Read the model definition and answer for the solid it produces. Units are mm, in the model's axes. A direction names the side the tool comes from. Round coordinates to 2 decimals unless told otherwise and drop trailing zeros. Order: outer loops, then holes, each group sorted by start corner. A loop starts at its lowest first (then second) coordinate and runs counter-clockwise, first axis right, second up. Notation, with made-up numbers: (18, 86) - (69, 86) arc R31 cw to (69, 120) - close; hole circle Ø2 at (57, 27.25). An arc over 180 degrees is marked (long way). Put each result on its own line as item: value. Start each with the question number.
Q1. Section A-A on x = -13.5 is taken. Give the vertices of the cut face in (y, z), then the cut area to 3 significant figures.
Q2. Find the intervals of material crossed by line 1 along Y through (x, z) = (0, 15.25); line 2 along Z through (x, y) = (14, 17); line 3 along X through (y, z) = (20, 13.75), in increasing order. Write a range as from..to.
Q3. Each of these flat-tipped pins is pushed along its axis until it touches: pin 1 Ø1.2 at (x, y) = (-6.93, -4) entering from -Z; pin 2 Ø25 at (x, y) = (11, 6.5) entering from -Z; pin 3 Ø1.5 at (x, z) = (17.5, 10.5) entering from +Y; pin 4 Ø6.5 at (x, y) = (0, 0) entering from -Z. Where does it stop, or does it pass through?
Q4. Section D-D on x = 18 is taken. Give the vertices of the cut face in (y, z).
Q5. Which of the six approach directions +Z, -Z, +X, -X, +Y, -Y give full straight-line access (tool end or side, diameter ignored) to faces 1 (the face through (-24, -24, 3)), 2 (the face through (-1.172, 8.923, 2.493)), 3 (the face through (24, -24, 14.5))?
Q6. For a pull along Y with two mould halves and no side action, classify faces 4 (the face through (0, 6, 14.5)), 5 (the face through (-11.5, 0.4, 0)), 6 (the face through (0, -25, 1)), 7 (the face through (-24, 24, 0)) as pulls with the +Y half, pulls with the -Y half, needs draft (parallel to the pull), parting line crosses it, or undercut.
Q7. Section B-B on z = 16.5 is taken. Give the vertices of the cut face in (x, y), then the cut area to 3 significant figures.
from build123d import *

# Parameters (mm, degrees)
SKETCH_W          = 50
SKETCH_H          = 50
SKETCH_R          = 9
PAD_DEPTH         = 3
SKETCH001_R       = 4
PAD001_DEPTH      = 1
PAD001_DEPTH_BACK = 14.5
SKETCH002_W       = 50
SKETCH002_H       = 50
SKETCH002_R       = 1
SKETCH002_R_2     = 3
SKETCH002_R_3     = 2
PAD002_DEPTH      = 3
FILLET_R          = 2


with BuildPart() as part:
    # Sketch → Pad (new body)
    with BuildSketch(Plane.XY):
        Rectangle(SKETCH_W, SKETCH_H)
        Circle(SKETCH_R, mode=Mode.SUBTRACT)
    extrude(amount=PAD_DEPTH)

    # Sketch001 (on Face6 of Pad) → Pad001 (join, two sides)
    with BuildSketch(Plane(origin=(0, 0, 0), x_dir=(1, 0, 0), z_dir=(0, 0, -1))) as pad001_sk:
        with Locations((-21, 21)):
            Circle(SKETCH001_R)
        with Locations((21, 21)):
            Circle(SKETCH001_R)
        with Locations((21, -21)):
            Circle(SKETCH001_R)
        with Locations((-21, -21)):
            Circle(SKETCH001_R)
    extrude(amount=PAD001_DEPTH)
    extrude(pad001_sk.sketch, amount=-PAD001_DEPTH_BACK)

    # Sketch002 (on Face25 of Pad001) → Pad002 (join)
    with BuildSketch(Plane.XY.offset(14.5)):
        Rectangle(SKETCH002_W, SKETCH002_H)
        with Locations((0, 8)):
            Circle(SKETCH002_R, mode=Mode.SUBTRACT)
        with Locations((6.928203, -4)):
            Circle(SKETCH002_R, mode=Mode.SUBTRACT)
        with Locations((-6.928203, -4)):
            Circle(SKETCH002_R, mode=Mode.SUBTRACT)
        with Locations((0, -8)):
            Circle(SKETCH002_R_2, mode=Mode.SUBTRACT)
        Circle(SKETCH002_R_3, mode=Mode.SUBTRACT)
    extrude(amount=PAD002_DEPTH)

    # Fillet
    fillet_edges = [part.edges().sort_by_distance(p)[0] for p in [
        (-9, 0, 0),
    ]]
    fillet(fillet_edges, radius=FILLET_R)


solid = part.part
Findings:
1. outline: (-25, 0) - (25, 0) - (25, 3) - (-25, 3) - close; (-25, 14.5) - (25, 14.5) - (25, 17.5) - (-25, 17.5) - close
1. area: 300 mm2
2. line 1: -25..-11, -5..-2, 2..7, 9..25
2. line 2: 0..3, 14.5..17.5
2. line 3: -24.87..-17.13, 17.13..24.87
3. pin 1: through
3. pin 2: z = 0
3. pin 3: y = 23.9
3. pin 4: z = 14.5
4. outline: (-25, 0) - (-23.65, 0) - (-23.65, -1) - (-18.35, -1) - (-18.35, 0) - (18.35, 0) - (18.35, -1) - (23.65, -1) - (23.65, 0) - (25, 0) - (25, 3) - (23.65, 3) - (23.65, 14.5) - (25, 14.5) - (25, 17.5) - (-25, 17.5) - (-25, 14.5) - (-23.65, 14.5) - (-23.65, 3) - (-25, 3) - close; hole (-18.35, 3) - (18.35, 3) - (18.35, 14.5) - (-18.35, 14.5) - close
5. face 1: -X, -Y
5. face 2: -Z
5. face 3: +X, -Y
6. face 4: undercut
6. face 5: undercut
6. face 6: pulls with the -Y half
6. face 7: needs draft
7. outline: (-25, -25) - (25, -25) - (25, 25) - (-25, 25) - close; hole circle Ø2 at (-6.93, -4); hole circle Ø6 at (0, -8); hole circle Ø4 at (0, 0); hole circle Ø2 at (0, 8); hole circle Ø2 at (6.93, -4)
7. area: 2,450 mm2
